Drawing for the job (mm, zero at the part's lowest x, y, z). A direction names the side the tool comes from. Coordinates: 2 decimals unless noted, no trailing zeros. Write each loop counter-clockwise with the first axis right and the second up, starting at its lowest first coordinate (ties: lowest second). Pieces come first, ordered by that corner, then holes. Notation, with made-up numbers: (10, 54) -> (30, 54) arc R5 cw to (30, 61) -> close; hole circle Ø9 at (-30, -5.75). An arc over 180 degrees is marked (long way). Write item = value, one per line. Start each with the question number.
Q1. Pull direction X, two halves, no side cores. Call the marked faces 4, 5 and 6: released by +X, released by -X, zero draft, split by the parting line, or undercut.
Q2. Pin check, flat tips, straight feed: P1, Ø2, axis at x = 8.5, y = 13, coming from the -Z side; P2, Ø3, axis at y = 9, z = 6, coming from the -X side; P3, Ø1.5, axis at x = 9.5, y = 8.5, coming from the +Z side; P4, Ø1.5, axis at y = 16, z = 64.5, coming from the -X side. Stop position of each tip, or through.
Q3. Band-saw the part on A-A, the plane y = 9. Give the number of separate pieces and of enclosed holes in the cut face, plus the area to 3 significant figures.
Q4. Band-saw the part on B-B, the plane z = 6. List the corners of the cut face in (x, y).
Q5. Probe line 1 (Z direction, x = 16.5, y = 9); line 2 (Z direction, x = 16.75, y = 14.25); line 3 (Z direction, x = 2.25, y = 12.5). List the from-to ranges inside material, lowest first.
Q6. Band-saw the part on C-C, the plane x = 9. List the corners of the cut face in (y, z), plus the area to 3 significant figures.
Q7. Tool access for the marked faces 1, 2 and 3: list every direction of +Z, -Z, +X, -X, +Y, -Y with a clear straight run to the whole face (end or side of a thin tool).
Q8. Band-saw the part on D-D, the plane z = 20. List the corners of the cut face in (x, y).
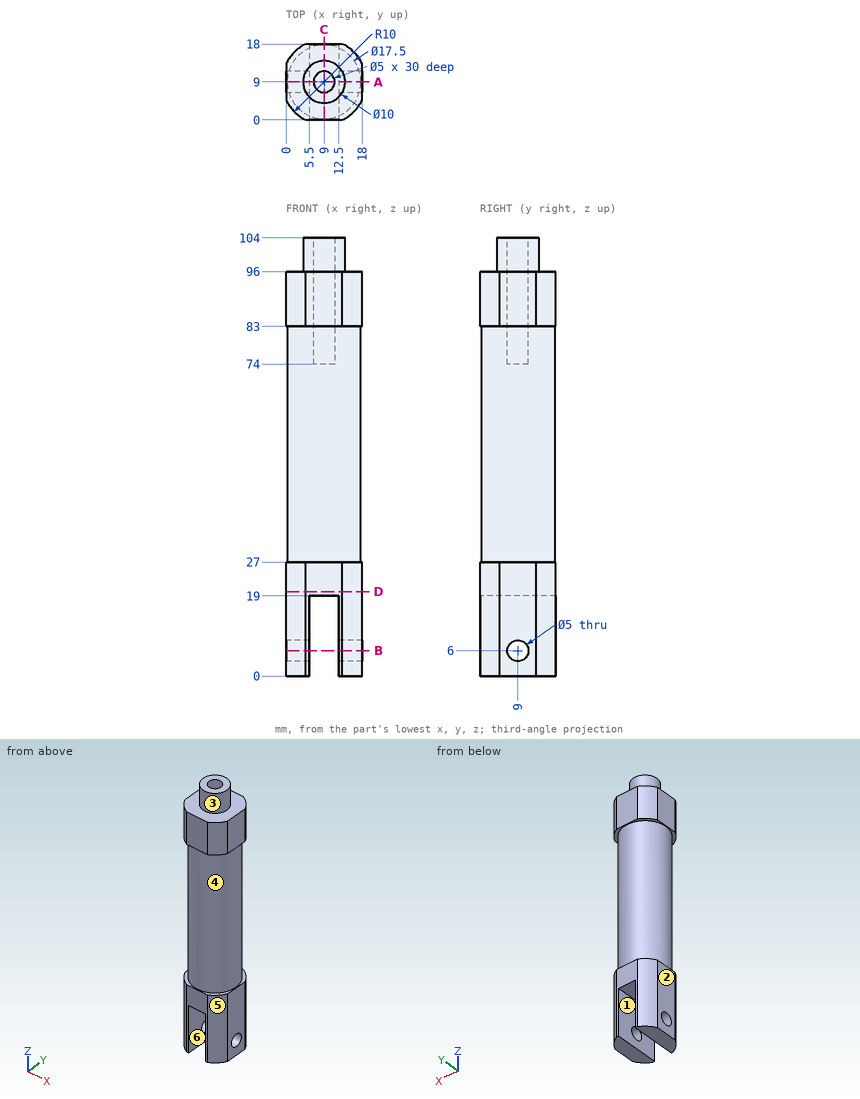
Ans:
q1.face_4 = split by the parting line
q1.face_5 = released by +X
q1.face_6 = undercut
q2.P1 = 19
q2.P2 = through
q2.P3 = 74
q2.P4 = 2.88
q3.separate_pieces = 3
q3.enclosed_holes = 0
q3.area = 1,440 mm2
q4.outline = (0, 4.64) arc R10 ccw to (4.64, 0) -> (5.5, 0) -> (5.5, 6.5) -> (0, 6.5) -> close; (0, 11.5) -> (5.5, 11.5) -> (5.5, 18) -> (4.64, 18) arc R10 ccw to (0, 13.36) -> close; (12.5, 0) -> (13.36, 0) arc R10 ccw to (18, 4.64) -> (18, 6.5) -> (12.5, 6.5) -> close; (12.5, 11.5) -> (18, 11.5) -> (18, 13.36) arc R10 ccw to (13.36, 18) -> (12.5, 18) -> close
q5.line_1 = 0 to 3.5, 8.5 to 96
q5.line_2 = 0 to 27, 83 to 96
q5.line_3 = 0 to 96
q6.outline = (0, 19) -> (18, 19) -> (18, 27) -> (17.75, 27) -> (17.75, 83) -> (18, 83) -> (18, 96) -> (14, 96) -> (14, 104) -> (11.5, 104) -> (11.5, 74) -> (6.5, 74) -> (6.5, 104) -> (4, 104) -> (4, 96) -> (0, 96) -> (0, 83) -> (0.25, 83) -> (0.25, 27) -> (0, 27) -> close
q6.area = 1,290 mm2
q7.face_1 = -Z, +Y, -Y
q7.face_2 = +Z, -Z, -X, +Y, -Y
q7.face_3 = +Z
q8.outline = (0, 4.64) arc R10 ccw to (4.64, 0) -> (13.36, 0) arc R10 ccw to (18, 4.64) -> (18, 13.36) arc R10 ccw to (13.36, 18) -> (4.64, 18) arc R10 ccw to (0, 13.36) -> close
